Geometry check sheet. Reference: drawing and pictorial views, mm from the part's lowest x, y, z. A direction names the side the tool comes from. Round coordinates to 2 decimals unless told otherwise and drop trailing zeros. Order: outer loops, then holes, each group sorted by start corner. A loop starts at its lowest first (then second) coordinate and runs counter-clockwise, first axis right, second up.
(1) Sectioned sample at B-B (x = 20). Record the boundary of the cut face in (y, z).
(2) Material ranges on line 1 along Y through (x, z) = (3, 1.7); line 2 along X through (y, z) = (5.75, 5.25); line 3 along X through (y, z) = (2.8, 3), recorded low to high.
(3) Release check for a two-part mould opening along Y. For the marked faces 3, 4 and 5 record: +Y half, -Y half, draft (parallel to the pull), parting line (faces both ways), or undercut.
(4) Go/stop test with flat-tipped pins: pin 1 (4 mm diameter, centred on x = 28.75, z = 5, fed in from +Y); pin 2 (3 mm diameter, centred on y = 2.5, z = 8.5, fed in from +X); pin 3 (1.5 mm diameter, centred on y = 0.5, z = 8.5, fed in from +X). Record where each tip stops, or that it passes through.
(5) Set-up check for the marked faces 1 and 2: record each of +Z, -Z, +X, -X, +Y, -Y from which the full face is reachable in a straight line by a thin tool's end or side.
(6) Sectioned sample at A-A (y = 3). Give the number of separate pieces and of enclosed holes in the cut face, plus the area to 3 significant figures.
(7) Sectioned sample at D-D (z = 13.75). Record the boundary of the cut face in (x, y).
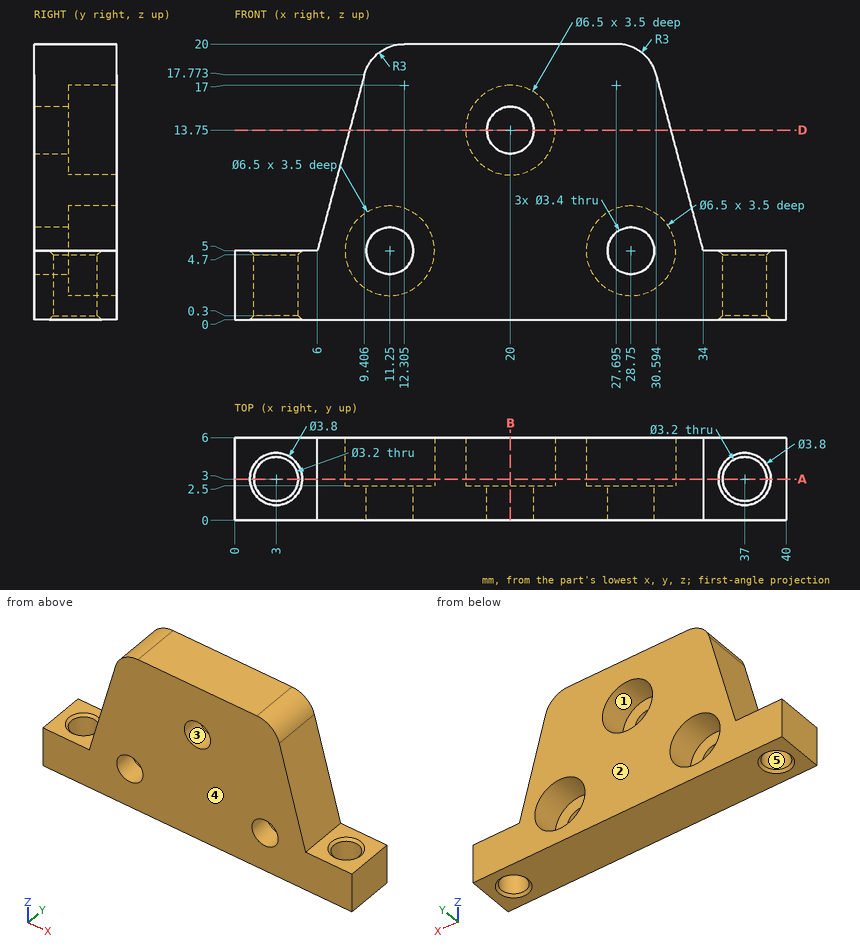
Answer below:
1. outline: (0, 0) - (6, 0) - (6, 10.5) - (2.5, 10.5) - (2.5, 12.05) - (0, 12.05) - close; (0, 15.45) - (2.5, 15.45) - (2.5, 17) - (6, 17) - (6, 20) - (0, 20) - close
2. line 1: y = 0 to 1.4, 4.6 to 6
2. line 2: x = 6.07 to 8.01, 14.49 to 25.51, 31.99 to 33.93
2. line 3: x = 0 to 1.41, 4.59 to 8.69, 13.81 to 26.19, 31.31 to 35.41, 38.59 to 40
3. face 3: draft
3. face 4: -Y half
3. face 5: undercut
4. pin 1: stops at y = 2.5
4. pin 2: stops at x = 33.47
4. pin 3: stops at x = 33.27
5. face 1: +Y
5. face 2: +Z, -Z, +X, -X, +Y
6. separate pieces: 3
6. enclosed holes: 3
6. area: 426 mm2
7. outline: (8.33, 0) - (18.3, 0) - (18.3, 2.5) - (16.75, 2.5) - (16.75, 6) - (8.33, 6) - close; (21.7, 0) - (31.67, 0) - (31.67, 6) - (23.25, 6) - (23.25, 2.5) - (21.7, 2.5) - close
